```python
from build123d import *

# Parameters (mm, degrees)
SKETCH_1_R      = 1.75
EXTRUDE_1_DEPTH = 3


with BuildPart() as part:
    # Sketch 1 → Extrude 1 (new body)
    with BuildSketch(Plane(origin=(0, 0, 0), x_dir=(1, 0, 0), z_dir=(0, 1, 0))):
        with BuildLine():
            Line((-56, 57), (-56, 45))
            Line((-56, 45), (28, 45))
            Line((28, 45), (28, 57))
            Line((28, 57), (73, 57))
            ThreePointArc((73, 57), (75.121320344, 56.121320344), (76, 54))
            Line((76, 54), (76, 47))
            Line((76, 47), (67, 47))
            Line((67, 47), (67, -33))
            Line((67, -33), (76, -33))
            Line((76, -33), (76, -54))
            ThreePointArc((76, -54), (75.121320344, -56.121320344), (73, -57))
            Line((73, -57), (-73, -57))
            ThreePointArc((-73, -57), (-75.121320344, -56.121320344), (-76, -54))
            Line((-76, -54), (-76, -18))
            Line((-76, -18), (-58, -18))
            Line((-58, -18), (-58, 27))
            Line((-58, 27), (-76, 27))
            Line((-76, 27), (-76, 54))
            ThreePointArc((-76, 54), (-75.121320344, 56.121320344), (-73, 57))
            Line((-73, 57), (-56, 57))
        make_face()
        with Locations(Location((-71, 52, 0), (0, 0, 270))):
            Circle(SKETCH_1_R, mode=Mode.SUBTRACT)
        with Locations(Location((71, 52, 0), (0, 0, 270))):
            Circle(SKETCH_1_R, mode=Mode.SUBTRACT)
        with Locations(Location((71, -52, 0), (0, 0, 270))):
            Circle(SKETCH_1_R, mode=Mode.SUBTRACT)
        with Locations(Location((-71, -52, 0), (0, 0, 270))):
            Circle(SKETCH_1_R, mode=Mode.SUBTRACT)
        with Locations(Location((-71, 40, 0), (0, 0, 270))):
            Circle(SKETCH_1_R, mode=Mode.SUBTRACT)
        with Locations(Location((71, -42, 0), (0, 0, 270))):
            Circle(SKETCH_1_R, mode=Mode.SUBTRACT)
        with Locations(Location((-71, -42, 0), (0, 0, 270))):
            Circle(SKETCH_1_R, mode=Mode.SUBTRACT)
    extrude(amount=EXTRUDE_1_DEPTH)


solid = part.part
```
The model under review builds one solid part; all positions refer to its coordinate system, in mm. A direction names the side the tool comes from. Round coordinates to 2 decimals unless told otherwise and drop trailing zeros. Write each loop counter-clockwise with the first axis right and the second up, starting at its lowest first coordinate (ties: lowest second). Pieces come first, ordered by that corner, then holes.
(1) We need section C-C on x = 71. Give the boundary of the cut face in (y, z).
(2) Mouldability with a two-part tool opening along X and no side actions: class faces 6 (the flat face through (-67, 1, 18)), 7 (the flat face through (-15, 1, -45)), 8 (the flat face through (-76, 1, 36)) as +X half, -X half, draft (parallel to the pull), parting line (faces both ways), or undercut.
(3) Wall thickness on L1, parallel to X at y = 2.15, z = 42; L2, parallel to Z at x = 71, y = 1.4; L3, parallel to X at y = 1.2, z = -52: over which ranges is each line inside the solid? List them lowest first.
(4) We need section B-B on x = -71. Give the boundary of the cut face in (y, z), and give its area (3 significant figures).
(5) Insertion check: pin 1 (3 mm diameter, centred on x = -71, z = -40, fed in from +Y); pin 2 (0.9 mm diameter, centred on x = 2, y = 1.5, fed in from -Z). Each pin has a flat end and moves straight along its axis. Give the tip position at first contact, or say it passes through.
(6) We need section D-D on y = 1.55. Give the boundary of the cut face in (x, z).
(7) Machinability: for faces 1 (the flat face through (71, 1, 33)), 2 (the cylindrical face through (-71.67, 1.479, 53.617)), 3 (the flat face through (28, 1, -51)), 4 (the flat face through (-58, 1, -4)), 5 (the flat face through (-76, 1, -40)), which of the approach directions +Z, -Z, +X, -X, +Y, -Y give a long, thin tool a straight path to every point of the face, cutting with its end or side? Answer none if there is none.
(8) We need section A-A on z = -40. Give the boundary of the cut face in (x, y), and give its area (4 significant figures).
Findings below:
1. outline: (0, -57) - (3, -57) - (3, -53.75) - (0, -53.75) - close; (0, -50.25) - (3, -50.25) - (3, -47) - (0, -47) - close; (0, 33) - (3, 33) - (3, 40.25) - (0, 40.25) - close; (0, 43.75) - (3, 43.75) - (3, 50.25) - (0, 50.25) - close; (0, 53.75) - (3, 53.75) - (3, 57) - (0, 57) - close
2. face 6: draft
2. face 7: undercut
2. face 8: -X half
3. L1: x = -76 to -72.75, -69.25 to 69.25, 72.75 to 76
3. L2: z = -57 to -53.75, -50.25 to -47, 33 to 40.25, 43.75 to 50.25, 53.75 to 57
3. L3: x = -76 to -72.75, -69.25 to -56, 28 to 69.25, 72.75 to 76
4. outline: (0, -57) - (3, -57) - (3, -53.75) - (0, -53.75) - close; (0, -50.25) - (3, -50.25) - (3, -41.75) - (0, -41.75) - close; (0, -38.25) - (3, -38.25) - (3, -27) - (0, -27) - close; (0, 18) - (3, 18) - (3, 40.25) - (0, 40.25) - close; (0, 43.75) - (3, 43.75) - (3, 50.25) - (0, 50.25) - close; (0, 53.75) - (3, 53.75) - (3, 57) - (0, 57) - close
4. area: 165 mm2
5. pin 1: passes through
5. pin 2: stops at z = -45
6. outline: (-76, -54) arc R3 ccw to (-73, -57) - (-56, -57) - (-56, -45) - (28, -45) - (28, -57) - (73, -57) arc R3 ccw to (76, -54) - (76, -47) - (67, -47) - (67, 33) - (76, 33) - (76, 54) arc R3 ccw to (73, 57) - (-73, 57) arc R3 ccw to (-76, 54) - (-76, 18) - (-58, 18) - (-58, -27) - (-76, -27) - close; hole circle Ø3.5 at (-71, -52); hole circle Ø3.5 at (-71, -40); hole circle Ø3.5 at (-71, 42); hole circle Ø3.5 at (-71, 52); hole circle Ø3.5 at (71, -52); hole circle Ø3.5 at (71, 42); hole circle Ø3.5 at (71, 52)
7. face 1: +X, +Y, -Y
7. face 2: +Y, -Y
7. face 3: -Z, +Y, -Y
7. face 4: -X, +Y, -Y
7. face 5: +Z, -Z, -X, +Y, -Y
8. outline: (-76, 0) - (-72.75, 0) - (-72.75, 3) - (-76, 3) - close; (-69.25, 0) - (67, 0) - (67, 3) - (-69.25, 3) - close
8. area: 418.5 mm2
